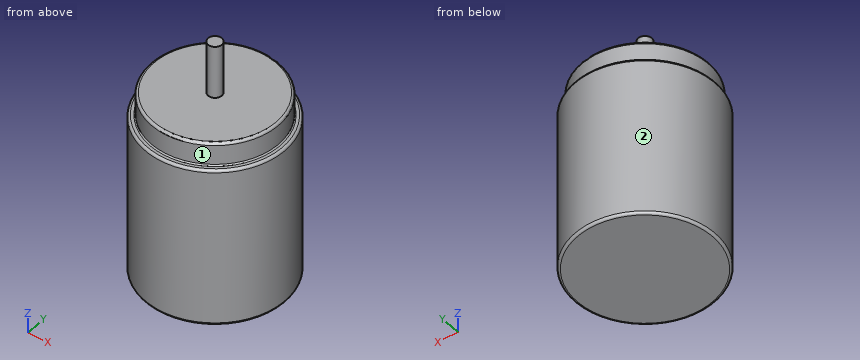
Autodesk Inventor part; units mm, degrees
ref_plane "YZ Plane" through (0, 0, 0) normal (1, 0, 0) x (0, 1, 0)
ref_plane "XZ Plane" through (0, 0, 0) normal (0, 1, 0) x (-1, 0, 0)
ref_plane "XY Plane" through (0, 0, 0) normal (0, 0, 1) x (1, 0, 0)
sketch "Sketch1" plane through (0, 0, 0) normal (0, 0, 1) x (1, 0, 0)
  circle A0 centre (0, 0) radius 1.016
  circle A1 centre (0, 0) radius 10.414
  dimension "d0" = 2.032
  dimension "d1" = 20.828
extrude "Extrusion1" add sketch "Sketch1" along normal blind 7.874 contours A0
extrude "Extrusion2" add sketch "Sketch1" against normal blind 27.305 contours A0 | A1
sketch "Sketch2" plane through (0, 0, 0) normal (0, 0, 1) x (1, 0, 0)
  circle A0 centre (0, 0) radius 9.4615
  circle A1 centre (0, 0) radius 10.414
  dimension "d6" = 18.923
extrude "Extrusion3" cut sketch "Sketch2" against normal blind 3.429
fillet "Fillet1" radius 0.3556 3 edges at (-9.4615, 0, 0) (-10.414, 0, -3.429) (-10.414, 0, -27.305)
fillet "Fillet2" radius 0.1778 1 edges at (-9.4615, 0, -3.429)
properties part number "Motor"
Input: part model. Units: mm. Frame: model coordinates. Face numbers are marked on the shaded views. A direction names the side the tool comes from. Give positions to 0.01 mm unless a question says otherwise; leave off trailing zeros. Order: outer loops, then holes, each group sorted by start corner. A loop starts at its lowest first (then second) coordinate and runs counter-clockwise, first axis right, second up. Notation, with made-up numbers: (32.5, 19.25) - (72.5, 19.25) arc R15 ccw to (72.5, 32.25) - close; hole circle Ø9 at (31.5, -29). An arc over 180 degrees is marked (long way). Use a Markdown table: item, result.
(1) Access query for the marked faces 1 and 2. Directions: +Z, -Z, +X, -X, +Y, -Y. A direction counts if a zero-diameter tool reaches every point of the face in a straight line with its end or side. Return the directions, or none.
Computed values:
| item | result |
|---|---|
| face 1 | +Z |
| face 2 | +Z, -Z |
(2) Line query: line 1 (Z direction, x = -3.5, y = 3) (3 decimals); line 2 (Y direction, x = 1.5, z = -7.5); line 3 (Y direction, x = 0.75, z = -15). Output: solid intervals per line, ascending. Write a range as from..to.
Computed values:
| item | result |
|---|---|
| line 1 | z = -27.305..0 |
| line 2 | y = -10.31..10.31 |
| line 3 | y = -10.39..10.39 |
(3) Section query C-C (z = -1). Output: boundary loops of the cut face in (x, y), then the cut area to 3 significant figures.
Computed values:
| item | result |
|---|---|
| outline | circle Ø18.92 at (0, 0) |
| area | 281 mm2 |
(4) Pin query (flat end, axial travel): pin 1 (2 mm diameter, centred on x = 1, y = -8, fed in from +Z); pin 2 (10 mm diameter, centred on x = -3, z = -12, fed in from +Y); pin 3 (1.5 mm diameter, centred on x = -4, z = -3.5, fed in from +Y); pin 4 (5 mm diameter, centred on y = 5.5, z = -13, fed in from +X). Return the tip coordinate at first contact, or that it passes through.
Computed values:
| item | result |
|---|---|
| pin 1 | stops at z = 0 |
| pin 2 | stops at y = 10.41 |
| pin 3 | stops at y = 9.88 |
| pin 4 | stops at x = 9.97 |
(5) Section query D-D (z = -12). Output: boundary loops of the cut face in (x, y), then the cut area to 3 significant figures.
Computed values:
| item | result |
|---|---|
| outline | circle Ø20.83 at (0, 0) |
| area | 341 mm2 |
